Input: part model. Units: mm. Frame: model coordinates. Face numbers are marked on the shaded views. A direction names the side the tool comes from. Coordinates: 2 decimals unless noted, no trailing zeros. Loops run counter-clockwise (first coordinate to the right, second up) from the corner with the lowest first, then second, coordinate; pieces in that order, holes last. Notation, with made-up numbers: M -0.5,-38 L 32.5,-38 A14 ccw 32.5,-13 Z; hole C 9.25,-16 d8. An arc over 180 degrees is marked long. Use a Markdown table: item, result. Add a question column.
1. Set-up query: the marked faces 1 and 2. Return all of +Z, -Z, +X, -X, +Y, -Y with unobstructed straight access to the full face (end or side cutting, diameter ignored); none if empty.
2. Section A-A on x = 0. Output: boundary loops of the cut face in (y, z).
3. Line query: L1, parallel to X at y = -3, z = 9.5; L2, parallel to X at y = -27.55, z = 7.5; L3, parallel to X at y = 23.5, z = 1. Output: solid intervals per line, ascending. Write a range as [from, to].
4. Pin query (flat end, axial travel): pin 1 (6 mm diameter, centred on y = 11, z = 9.5, fed in from +X); pin 2 (2.5 mm diameter, centred on x = 16.5, y = -27.5, fed in from +Z); pin 3 (4.5 mm diameter, centred on x = 18, z = 7.5, fed in from +Y). Return the tip coordinate at first contact, or that it passes through.
5. Section C-C on z = 13.75. Output: boundary loops of the cut face in (x, y) (3 decimals), then the cut area to 3 significant figures.
6. Section B-B on y = -27. Output: boundary loops of the cut face in (x, z), then the cut area to 3 significant figures.
7. Section D-D on z = 8.5. State how many separate pieces and enclosed holes the cut face has, then the cut area to 3 significant figures.
8. Draft query along X for the marked faces 3, 4, 5 and 6. Return one class per face: +X half, -X half, draft (parallel to the pull), parting line (faces both ways), or undercut.
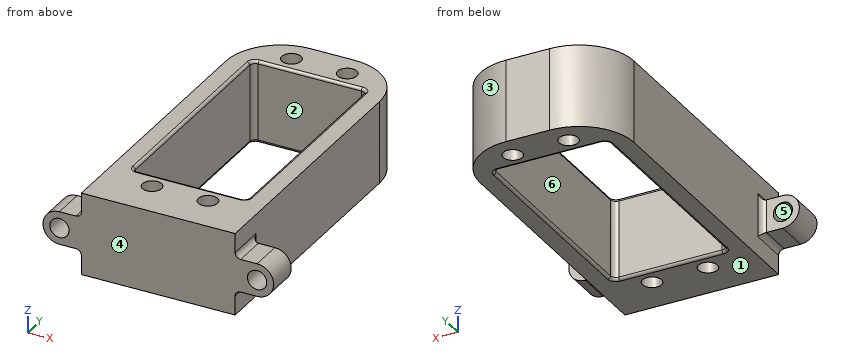
```python
from build123d import *

# Parameters (mm, degrees)
SKETCH1_W           = 28
SKETCH1_H           = 56
SKETCH1_R           = 1.75
SKETCH1_W_2         = 20.8
SKETCH1_H_2         = 40.8
BOSS_EXTRUDE1_DEPTH = 15
FILLET1_R           = 10
FILLET2_R           = 1
FILLET3_R           = 0.5
SKETCH2_R           = 3
SKETCH2_R_2         = 1.75
BOSS_EXTRUDE2_DEPTH = 3
FILLET4_R           = 1
FILLET5_R           = 1
BOSS_EXTRUDE3_START = 3
SKETCH3_R           = 1.75
BOSS_EXTRUDE3_DEPTH = 3


with BuildPart() as part:
    # Sketch1 → Boss-Extrude1 (new body)
    with BuildSketch(Plane.XY):
        Rectangle(SKETCH1_W, SKETCH1_H)
        with Locations((-5.085, 23.63)):
            Circle(SKETCH1_R, mode=Mode.SUBTRACT)
        with Locations((5.085, 23.63)):
            Circle(SKETCH1_R, mode=Mode.SUBTRACT)
        with Locations((-5.085, -23.63)):
            Circle(SKETCH1_R, mode=Mode.SUBTRACT)
        with Locations((5.085, -23.63)):
            Circle(SKETCH1_R, mode=Mode.SUBTRACT)
        Rectangle(SKETCH1_W_2, SKETCH1_H_2, mode=Mode.SUBTRACT)
    extrude(amount=BOSS_EXTRUDE1_DEPTH)

    # Fillet1
    fillet1_edges = [part.edges().sort_by_distance(p)[0] for p in [
        (-14, 28, 7.5),
        (14, 28, 7.5),
    ]]
    fillet(fillet1_edges, radius=FILLET1_R)

    # Fillet2
    fillet2_edges = [part.edges().sort_by_distance(p)[0] for p in [
        (10.4, -20.4, 7.5),
        (10.4, 20.4, 7.5),
        (-10.4, 20.4, 7.5),
        (-10.4, -20.4, 7.5),
    ]]
    fillet(fillet2_edges, radius=FILLET2_R)

    # Fillet3
    fillet3_edges = [part.edges().sort_by_distance(p)[0] for p in [
        (0, -20.4, 0),
        (0, -20.4, 15),
        (10.4, 0, 0),
        (10.4, 0, 15),
        (-10.4, 0, 0),
        (-10.4, 0, 15),
        (0, 20.4, 0),
        (0, 20.4, 15),
        (10.107106781, -20.107106781, 0),
        (10.107106781, -20.107106781, 15),
        (-10.107106781, -20.107106781, 0),
        (-10.107106781, -20.107106781, 15),
        (-10.107106781, 20.107106781, 0),
        (-10.107106781, 20.107106781, 15),
        (10.107106781, 20.107106781, 0),
        (10.107106781, 20.107106781, 15),
    ]]
    fillet(fillet3_edges, radius=FILLET3_R)

    # Sketch2 → Boss-Extrude2 (add)
    # profile 1 of 4: a face of its own
    with BuildSketch(Plane.XZ.offset(28)):
        with Locations((-18, 7.5)):
            Circle(SKETCH2_R)
        with Locations(Location((-18, 7.5, 0), (0, 0, 270))):
            Circle(SKETCH2_R_2, mode=Mode.SUBTRACT)
    # profile 2 of 4: a face of its own
    with BuildSketch(Plane.XZ.offset(28)):
        with BuildLine():
            Line((-18, 4.5), (-14, 4.5))
            Line((-14, 4.5), (-14, 10.5))
            Line((-14, 10.5), (-18, 10.5))
            ThreePointArc((-18, 10.5), (-15.878679656, 9.621320344), (-15, 7.5))
            ThreePointArc((-15, 7.5), (-15.878679656, 5.378679656), (-18, 4.5))
        make_face()
    # profile 3 of 4: a face of its own
    with BuildSketch(Plane.XZ.offset(28)):
        with BuildLine():
            Line((14, 4.5), (18, 4.5))
            ThreePointArc((18, 4.5), (15, 7.5), (18, 10.5))
            Line((18, 10.5), (14, 10.5))
            Line((14, 10.5), (14, 4.5))
        make_face()
    # profile 4 of 4: a face of its own
    with BuildSketch(Plane.XZ.offset(28)):
        with Locations((18, 7.5)):
            Circle(SKETCH2_R)
        with Locations(Location((18, 7.5, 0), (0, 0, 270))):
            Circle(SKETCH2_R_2, mode=Mode.SUBTRACT)
    extrude(amount=-BOSS_EXTRUDE2_DEPTH)

    # Fillet4
    fillet4_edges = [part.edges().sort_by_distance(p)[0] for p in [
        (-14, -25, 7.5),
        (14, -25, 7.5),
    ]]
    fillet(fillet4_edges, radius=FILLET4_R)

    # Fillet5
    fillet5_edges = [part.edges().sort_by_distance(p)[0] for p in [
        (14, -26, 10.5),
        (14, -26, 4.5),
        (-14, -26, 4.5),
        (-14, -26, 10.5),
    ]]
    fillet(fillet5_edges, radius=FILLET5_R)

    # Sketch3 → Boss-Extrude3 (add)
    with BuildSketch(Plane.XZ.offset(28).offset(BOSS_EXTRUDE3_START)):
        with BuildLine():
            Line((-14, 0), (14, 0))
            Line((14, 0), (14, 3.5))
            ThreePointArc((14, 3.5), (14.292893219, 4.207106781), (15, 4.5))
            Line((15, 4.5), (18, 4.5))
            ThreePointArc((18, 4.5), (21, 7.5), (18, 10.5))
            Line((18, 10.5), (15, 10.5))
            ThreePointArc((15, 10.5), (14.292893219, 10.792893219), (14, 11.5))
            Line((14, 11.5), (14, 15))
            Line((14, 15), (-14, 15))
            Line((-14, 15), (-14, 11.5))
            ThreePointArc((-14, 11.5), (-14.292893219, 10.792893219), (-15, 10.5))
            Line((-15, 10.5), (-18, 10.5))
            ThreePointArc((-18, 10.5), (-21, 7.5), (-18, 4.5))
            Line((-18, 4.5), (-15, 4.5))
            ThreePointArc((-15, 4.5), (-14.292893219, 4.207106781), (-14, 3.5))
            Line((-14, 3.5), (-14, 0))
        make_face()
        with Locations(Location((18, 7.5, 0), (0, 0, 270))):
            Circle(SKETCH3_R, mode=Mode.SUBTRACT)
        with Locations(Location((-18, 7.5, 0), (0, 0, 270))):
            Circle(SKETCH3_R, mode=Mode.SUBTRACT)
    extrude(amount=-BOSS_EXTRUDE3_DEPTH)


solid = part.part
```
Answers below:
| question | item | result |
|---|---|---|
| 1 | face 1 | -Z, +X, -X, +Y, -Y |
| 1 | face 2 | +Z, -Z |
| 2 | outline | M -31,0 L -20.9,0 A0.5 ccw -20.4,0.5 L -20.4,14.5 A0.5 ccw -20.9,15 L -31,15 Z; M 20.4,0.5 A0.5 ccw 20.9,0 L 28,0 L 28,15 L 20.9,15 A0.5 ccw 20.4,14.5 Z |
| 3 | L1 | x = [-14, -10.4], [10.4, 14] |
| 3 | L2 | x = [-21, -19.75], [-16.25, 16.25], [19.75, 21] |
| 3 | L3 | x = [-12.35, -6.83], [-3.34, 3.34], [6.83, 12.35] |
| 4 | pin 1 | stops at x = 14 |
| 4 | pin 2 | stops at z = 10.5 |
| 4 | pin 3 | stops at y = -25 |
| 5 | outline | M -14,-31 L 14,-31 L 14,18 A10 ccw 4,28 L -4,28 A10 ccw -14,18 Z; hole M -10.4,-19.4 A1 ccw -9.4,-20.4 L 9.4,-20.4 A1 ccw 10.4,-19.4 L 10.4,19.4 A1 ccw 9.4,20.4 L -9.4,20.4 A1 ccw -10.4,19.4 Z; hole C -5.085,-23.63 d3.5; hole C -5.085,23.63 d3.5; hole C 5.085,-23.63 d3.5; hole C 5.085,23.63 d3.5 |
| 5 | area | 723 mm² |
| 6 | outline | M -18,4.5 L -15,4.5 A1 cw -14,3.5 L -14,0 L 14,0 L 14,3.5 A1 cw 15,4.5 L 18,4.5 A3 ccw 18,10.5 L 15,10.5 A1 cw 14,11.5 L 14,15 L -14,15 L -14,11.5 A1 cw -15,10.5 L -18,10.5 A3 ccw Z; hole C -18,7.5 d3.5; hole C 18,7.5 d3.5 |
| 6 | area | 478 mm² |
| 7 | separate pieces | 3 |
| 7 | enclosed holes | 5 |
| 7 | area | 771 mm² |
| 8 | face 3 | +X half |
| 8 | face 4 | draft |
| 8 | face 5 | undercut |
| 8 | face 6 | undercut |
